The model under review builds one solid part; all positions refer to its coordinate system, in mm. Round coordinates to 2 decimals unless told otherwise and drop trailing zeros. Write each loop counter-clockwise with the first axis right and the second up, starting at its lowest first coordinate (ties: lowest second). Pieces come first, ordered by that corner, then holes. Notation, with made-up numbers: (3, 26.25) - (29, 26.25) arc R19 ccw to (29, 39.25) - close; hole circle Ø5 at (72, 43). An arc over 180 degrees is marked (long way). Return JSON: item names as keys, results as strings.
from build123d import *

# Parameters (mm, degrees)
SKETCH1_W               = 88.9
SKETCH1_H               = 403.225
BOSS_EXTRUDE1_DEPTH     = 9.525
SKETCH2_R               = 4.7625
CUT_EXTRUDE1_DEPTH      = 1
CUT_EXTRUDE1_DEPTH_BACK = 20.05


with BuildPart() as part:
    # Sketch1 → Boss-Extrude1 (new body, symmetric)
    with BuildSketch(Plane.XY):
        Rectangle(SKETCH1_W, SKETCH1_H)
    extrude(amount=BOSS_EXTRUDE1_DEPTH, both=True)

    # Sketch2 → Cut-Extrude1 (cut, two sides)
    with BuildSketch(Plane.XY.offset(9.525)) as cut_extrude1_sk:
        with Locations((-9.525, 173.0375)):
            Circle(SKETCH2_R)
    extrude(amount=CUT_EXTRUDE1_DEPTH, mode=Mode.SUBTRACT)
    extrude(cut_extrude1_sk.sketch, amount=-CUT_EXTRUDE1_DEPTH_BACK, mode=Mode.SUBTRACT)


solid = part.part
(1) Add section A-A (x = -8.5). Write out the cut boundary in (y, z) (1 decimal), plus the area to 3 significant figures.
Filled in:
{"outline": "(-201.6, -9.5) - (168.4, -9.5) - (168.4, 9.5) - (-201.6, 9.5) - close; (177.7, -9.5) - (201.6, -9.5) - (201.6, 9.5) - (177.7, 9.5) - close", "area": "7,500 mm2"}
(2) Wall thickness on line 1 (X direction, y = 171.5, z = -5); line 2 (Y direction, x = -8, z = 8.25): over which ranges is each line inside the solid? List them lowest first.
Filled in:
{"line 1": "x = -44.45 to -14.03, -5.02 to 44.45", "line 2": "y = -201.61 to 168.53, 177.55 to 201.61"}
(3) Mouldability with a two-part tool opening along Y and no side actions: class faces 1 (the cylindrical face through (-10.56, 168.39, 0.13)), 2 (the flat face through (44.45, -3, 0)), 3 (the flat face through (-1, 201.612, 0)), 4 (the flat face through (-1, -201.612, 0)) as released by +Y, released by -Y, zero draft, split by the parting line, or undercut.
Filled in:
{"face 1": "undercut", "face 2": "zero draft", "face 3": "released by +Y", "face 4": "released by -Y"}
